from build123d import *

# Parameters (mm, degrees)
CUT_EXTRUDE_1_DEPTH      = 176.555606187
CUT_EXTRUDE_1_DEPTH_BACK = 176.555606187
PATTERN_CIRCULAR_1_COUNT = 4
PATTERN_CIRCULAR_1_ANGLE = 90


with BuildPart() as part:
    # 草图1 → 旋转1 (revolve)
    with BuildSketch(Plane(origin=(0, 0, 0), x_dir=(0, 0, -1), z_dir=(1, 0, 0)), mode=Mode.PRIVATE) as revolve_1_sk:
        Polygon((-11, -123), (0, -123), (-12.701705922, -101), (-23.701705922, -101), align=None)
    revolve(revolve_1_sk.sketch.rotate(Axis((0, 0, 0), (0, 0, -1)), 270), axis=Axis((0, 0, 0), (0, 0, -1)))

    # 草图2 → 切除-拉伸1 (cut, two sides: drawn at the far end of the back side and taken through both)
    with BuildSketch(Plane.XY.offset(-CUT_EXTRUDE_1_DEPTH_BACK)):
        Polygon((-891.013215652, -57), (-178.582733939, -57), (163.038782242, -57), (875.469263955, -57), (875.469263955, 1367.860963427), (-891.013215652, 1367.860963427), align=None)
    extrude(amount=CUT_EXTRUDE_1_DEPTH + CUT_EXTRUDE_1_DEPTH_BACK, mode=Mode.SUBTRACT)

    # 草图4 → Ø7.0 (7) 直径孔1 (revolve, cut)
    with BuildSketch(Plane(origin=(78.488852712, -78.488852712, 0), x_dir=(0, 1, 0), z_dir=(1, 0, 0))):
        Polygon((0, 0), (0, 12.103012167), (3.5, 10), (3.5, 0), align=None)
    hole_wizard_7_0_7_1 = revolve(axis=Axis((78.488852712, -78.488852712, -6.35), (0, 0, 1)), mode=Mode.SUBTRACT)

    # 阵列(圆周)1: Ø7.0 (7) 直径孔1 ×4 about axis
    pattern_circular_1_axis = Axis((0, 0, 0), (0, 0, -1))
    for i in range(1, PATTERN_CIRCULAR_1_COUNT):
        add(hole_wizard_7_0_7_1.rotate(pattern_circular_1_axis, i * PATTERN_CIRCULAR_1_ANGLE / (PATTERN_CIRCULAR_1_COUNT - 1)), mode=Mode.SUBTRACT)


solid = part.part
Build history of the part. All positions in model axes, mm. A direction names the side the tool comes from. Coordinates: 2 decimals unless noted, no trailing zeros. Write each loop counter-clockwise with the first axis right and the second up, starting at its lowest first coordinate (ties: lowest second). Pieces come first, ordered by that corner, then holes.
(1) 3-axis set-ups, long thin cutter, end or side, ignore diameter. For faces 1 (the cylindrical face through (29.18, -110.69, 7.98)), 2 (the flat face through (96, -57, 12)): which of +Z, -Z, +X, -X, +Y, -Y reach the whole face in a straight line?
(2) Pin check, flat tips, straight feed: pin 1 Ø6.5 at (x, y) = (78.49, -78.49) entering from -Z; pin 2 Ø12 at (y, z) = (-88.5, 3.5) entering from -X; pin 3 Ø8 at (x, z) = (44.5, 14.5) entering from +Y. Stop position of each tip, or through.
(3) Cut at A-A on z = 16. List the corners of the cut face in (x, y).
(4) Mould opens along Y. For faces 3 (the cylindrical face through (1.37, -100.99, 18.28)), 4 (the cylindrical face through (1.875, -122.986, 5.423)), 5 (the conical face through (-79.096, -78.462, 11.738)) say: pulls with the +Y half, pulls with the -Y half, needs draft (parallel to the pull), parting line crosses it, or undercut.
(5) Drill centre lines: line 1 (X direction, y = -61, z = 20.75); line 2 (X direction, y = -107, z = 10.75); line 3 (X direction, y = -77, z = 20). Where is each one in solid material? Low to high.
Working result:
1. face 1: -Z
1. face 2: +Z, -Z, +X, -X, +Y
2. pin 1: stops at z = 10.15
2. pin 2: stops at x = -91.23
2. pin 3: stops at y = -88.59
3. outline: (-99.12, -57) arc R114.34 ccw to (99.12, -57) - (83.38, -57) arc R101 cw to (-83.38, -57) - close
4. face 3: pulls with the +Y half
4. face 4: pulls with the -Y half
4. face 5: undercut
5. line 1: x = -86.83 to -80.5, 80.5 to 86.83
5. line 2: x = -60.66 to -30.97, -26.49 to 26.49, 30.97 to 60.66
5. line 3: x = -74.89 to -65.36, 65.36 to 74.89
